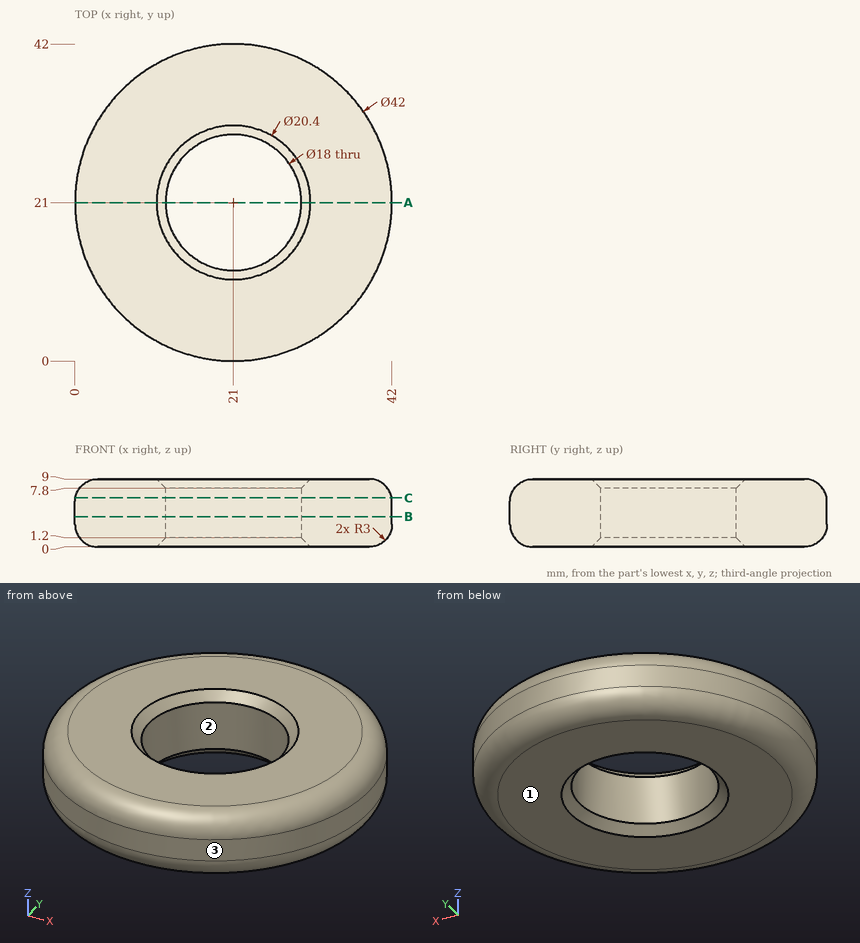
The figure shows three views and two pictorial views of one solid part (mm, origin at its lowest corner). Answer the questions. Round coordinates to 2 decimals unless told otherwise and drop trailing zeros. Order: outer loops, then holes, each group sorted by start corner. A loop starts at its lowest first (then second) coordinate and runs counter-clockwise, first axis right, second up. Notation, with made-up numbers: M 68.25,18.5 L 102.25,18.5 A30 cw 102.25,56.5 Z; hole C 80.25,61 d10. An arc over 180 degrees is marked long. Answer in a Markdown table with one row per item. Add a question column.
1) The part is cut by section A-A on y = 21. Determine the outline of the cut face in (x, z), plus the area to 3 significant figures.
2) Flat-ended cylindrical pins translate along their axes: pin 1 Ø2 at (x, y) = (11.5, 37.5) entering from -Z; pin 2 Ø1.5 at (y, z) = (7, 3) entering from +X; pin 3 Ø1.5 at (x, z) = (23, 7) entering from -Y. Find the tip coordinate at first contact, or state that the pin passes through.
3) The part is cut by section B-B on z = 4. Determine the outline of the cut face in (x, y).
4) The part is cut by section C-C on z = 6.5. Determine the outline of the cut face in (x, y).
5) Consider line 1 along Y through (x, z) = (21, 2.75); line 2 along X through (y, z) = (28.5, 0.5); line 3 along Y through (x, z) = (29, 5.5). Determine where each line is inside the solid, lowest interval first. Write a range as from..to.
6) Determine the mould class of the marked faces 1, 2 and 3 for opening direction Y: pulls with the +Y half, pulls with the -Y half, needs draft (parallel to the pull), parting line crosses it, or undercut.
Findings below:
| question | item | result |
|---|---|---|
| 1 | outline | M 0,3 A3 ccw 3,0 L 10.8,0 L 12,1.2 L 12,7.8 L 10.8,9 L 3,9 A3 ccw 0,6 Z; M 30,1.2 L 31.2,0 L 39,0 A3 ccw 42,3 L 42,6 A3 ccw 39,9 L 31.2,9 L 30,7.8 Z |
| 1 | area | 205 mm² |
| 2 | pin 1 | stops at z = 0 |
| 2 | pin 2 | stops at x = 37.29 |
| 2 | pin 3 | stops at y = 0.08 |
| 3 | outline | C 21,21 d42; hole C 21,21 d18 |
| 4 | outline | C 21,21 d41.92; hole C 21,21 d18 |
| 5 | line 1 | y = 0.01..12, 30..41.99 |
| 5 | line 2 | x = 2.83..14.85, 27.15..39.17 |
| 5 | line 3 | y = 1.58..16.88, 25.12..40.42 |
| 6 | face 1 | needs draft |
| 6 | face 2 | undercut |
| 6 | face 3 | parting line crosses it |
